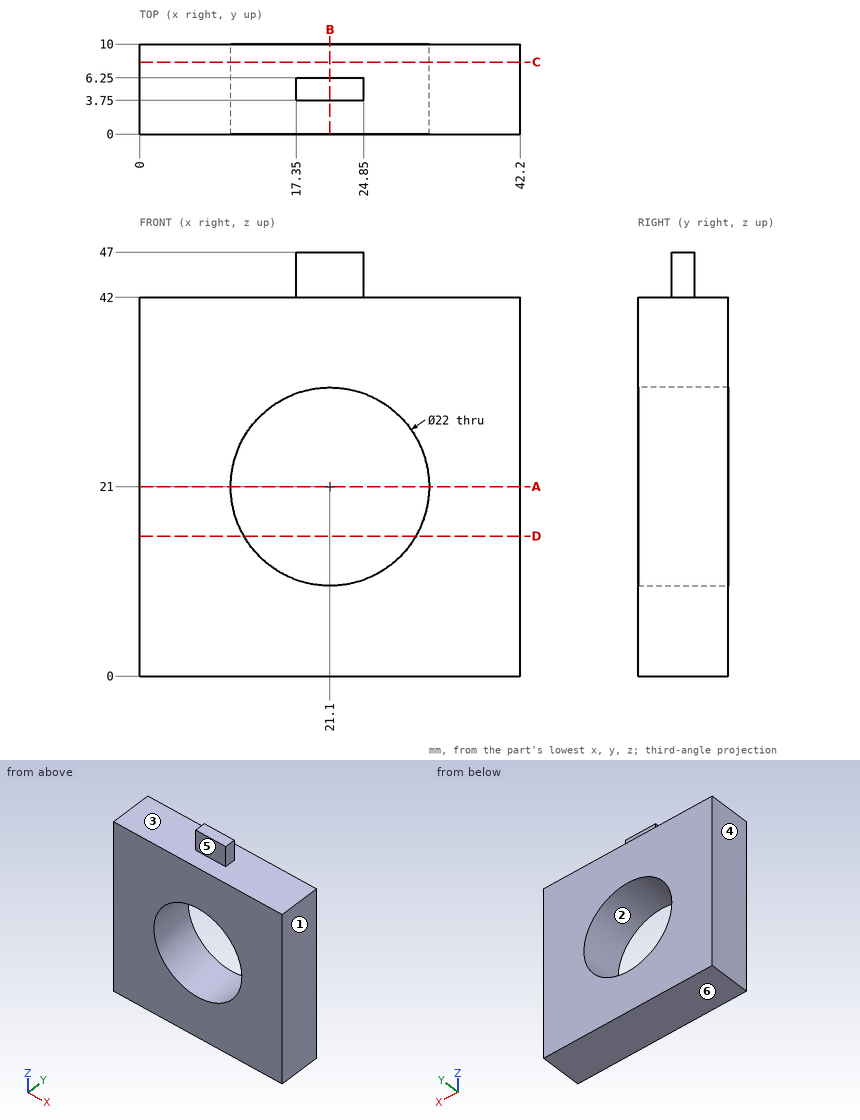
Here's the drawing with two shaded views (mm, measured from the low corner). I have some questions. A direction names the side the tool comes from. Give positions to 0.01 mm unless a question says otherwise; leave off trailing zeros. Loops run counter-clockwise (first coordinate to the right, second up) from the corner with the lowest first, then second, coordinate; pieces in that order, holes last. Notation, with made-up numbers: (-17, -9) -> (2, -9) arc R10 ccw to (2, 5) -> close; hole circle Ø11 at (8, 36). An arc over 180 degrees is marked (long way). Answer as a JSON object with one key per item and string values. Group by question number.
Item 1: I need wall thicknesses on L1, parallel to X at y = 4.5, z = 21; L2, parallel to X at y = 0.75, z = 18; L3, parallel to Z at x = 20.5, y = 2. Which ranges of each line are inside material? Lowest first, please.
Item 2: Imagine slicing it at D-D on z = 15.5. Write out the boundary of the cut face in (x, y), then the cut area to 3 significant figures.
Item 3: On a 3-axis mill with a long thin cutter (end or side, diameter ignored), from which of +Z, -Z, +X, -X, +Y, -Y can I reach the whole of each face in a straight line? I mean the marked faces 5 and 6. Say none if no direction works.
Item 4: Imagine slicing it at B-B on x = 21.1. Write out the boundary of the cut face in (y, z), then the cut area to 4 significant figures.
Item 5: Will these pins go through, and if not, where does the flat tip stop? pin 1 (1.2 mm diameter, centred on y = 5.5, z = 44.5, fed in from -X); pin 2 (2 mm diameter, centred on x = 35.5, y = 5, fed in from +Z); pin 3 (17.5 mm diameter, centred on x = 21.1, z = 21, fed in from +Y); pin 4 (1.5 mm diameter, centred on x = 22.5, z = 45.5, fed in from -Y).
Item 6: Thinking about a two-plate mould opening in X: for the marked faces 1, 2, 3 and 4, which applies, pulls with the +X half, pulls with the -X half, needs draft (parallel to the pull), parting line crosses it, or undercut?
Item 7: Imagine slicing it at A-A on z = 21. Write out the boundary of the cut face in (x, y).
Item 8: Imagine slicing it at C-C on y = 8. Write out the boundary of the cut face in (x, z), then the cut area to 3 significant figures.
Answer list:
{
 "1": {"L1": "x = 0 to 10.1, 32.1 to 42.2", "L2": "x = 0 to 10.52, 31.68 to 42.2", "L3": "z = 0 to 10.02, 31.98 to 42"},
 "2": {"outline": "(0, 0) -> (11.57, 0) -> (11.57, 10) -> (0, 10) -> close; (30.63, 0) -> (42.2, 0) -> (42.2, 10) -> (30.63, 10) -> close", "area": "231 mm2"},
 "3": {"face 5": "+Z, +X, -X, -Y", "face 6": "-Z, +X, -X, +Y, -Y"},
 "4": {"outline": "(0, 0) -> (10, 0) -> (10, 10) -> (0, 10) -> close; (0, 32) -> (10, 32) -> (10, 42) -> (6.25, 42) -> (6.25, 47) -> (3.75, 47) -> (3.75, 42) -> (0, 42) -> close", "area": "212.5 mm2"},
 "5": {"pin 1": "stops at x = 17.35", "pin 2": "stops at z = 42", "pin 3": "passes through", "pin 4": "stops at y = 3.75"},
 "6": {"face 1": "pulls with the +X half", "face 2": "undercut", "face 3": "needs draft", "face 4": "pulls with the -X half"},
 "7": {"outline": "(0, 0) -> (10.1, 0) -> (10.1, 10) -> (0, 10) -> close; (32.1, 0) -> (42.2, 0) -> (42.2, 10) -> (32.1, 10) -> close"},
 "8": {"outline": "(0, 0) -> (42.2, 0) -> (42.2, 42) -> (0, 42) -> close; hole circle Ø22 at (21.1, 21)", "area": "1,390 mm2"}
}
